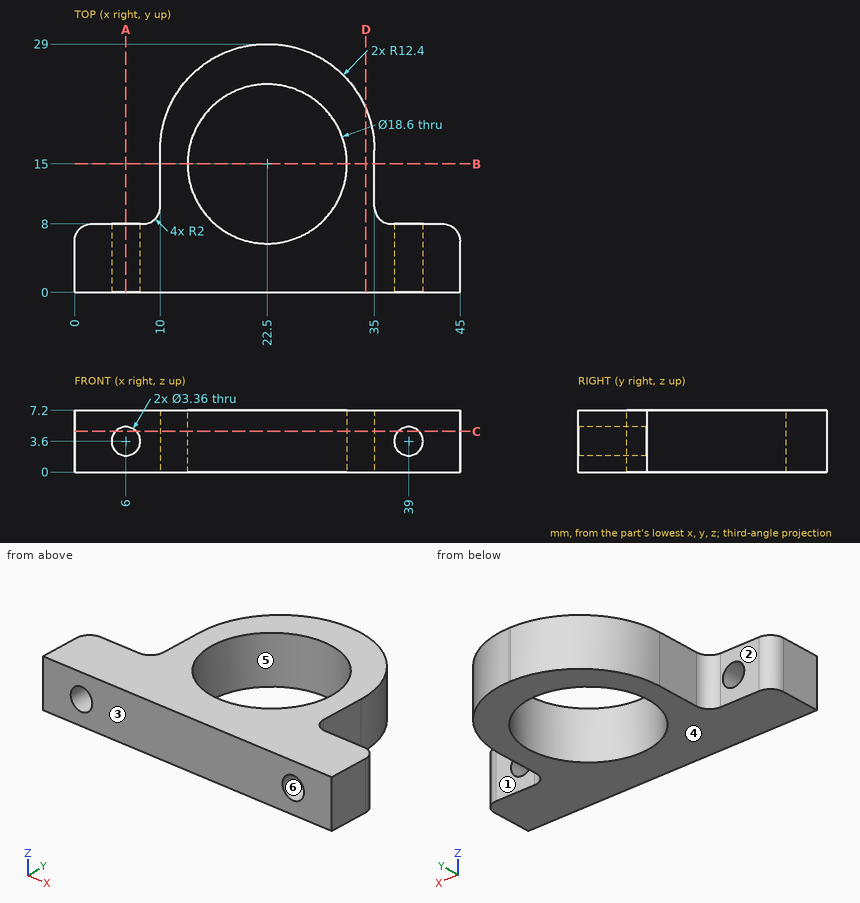
Drawing for the job (mm, zero at the part's lowest x, y, z). A direction names the side the tool comes from. Give positions to 0.01 mm unless a question says otherwise; leave off trailing zeros. Order: outer loops, then holes, each group sorted by start corner. A loop starts at its lowest first (then second) coordinate and runs counter-clockwise, first axis right, second up. Notation, with made-up numbers: (-9.5, -16) - (12.5, -16) arc R21 cw to (12.5, 1) - close; hole circle Ø2 at (-16, -38). An arc over 180 degrees is marked (long way). Use one line per item in the form item = value.
Item 1: Two-plate mould, pull along Z, no slides. Class the marked faces 4, 5 and 6: released by +Z, released by -Z, zero draft, split by the parting line, or undercut.
Solution:
face_4 = released by -Z
face_5 = zero draft
face_6 = undercut
Item 2: Slice it at D-D on x = 34. Give the cut face in (y, z).
Solution:
outline = (0, 0) - (21.48, 0) - (21.48, 7.2) - (0, 7.2) - close
Item 3: Probe probe 1 along Y at (x, z) = (22.5, 4); probe 2 along Z at (x, y) = (6, 3.75); probe 3 along X at (y, z) = (6.75, 4). List the from-to ranges inside material, lowest first. Write a range as from..to.
Solution:
probe_1 = 0..5.7, 24.3..29
probe_2 = 0..1.92, 5.28..7.2
probe_3 = 0.15..4.37, 7.63..18.21, 26.79..37.37, 40.63..44.85
Item 4: Slice it at B-B on y = 15. Give the cut face in (x, z).
Solution:
outline = (10, 0) - (13.2, 0) - (13.2, 7.2) - (10, 7.2) - close; (31.8, 0) - (35, 0) - (35, 7.2) - (31.8, 7.2) - close
Item 5: Pin check, flat tips, straight feed: pin 1 Ø3 at (x, z) = (4.5, 2.5) entering from +Y; pin 2 Ø2 at (x, z) = (37.5, 6) entering from +Y; pin 3 Ø2 at (y, z) = (20.5, 1.5) entering from -X; pin 4 Ø5 at (x, y) = (12, 25) entering from +Z. Stop position of each tip, or through.
Solution:
pin_1 = 8
pin_2 = 8.06
pin_3 = 10.34
pin_4 = 7.2
Item 6: Slice it at C-C on z = 4.75. Give the cut face in (x, y), and give its area (3 significant figures).
Solution:
outline = (0, 0) - (4.78, 0) - (4.78, 8) - (2, 8) arc R2 ccw to (0, 6) - close; (7.22, 0) - (37.78, 0) - (37.78, 8) - (37, 8) arc R2 cw to (35, 10) - (35, 16.6) arc R12.4 ccw to (22.6, 29) - (22.4, 29) arc R12.4 ccw to (10, 16.6) - (10, 10) arc R2 cw to (8, 8) - (7.22, 8) - close; (40.22, 0) - (45, 0) - (45, 6) arc R2 ccw to (43, 8) - (40.22, 8) - close; hole circle Ø18.6 at (22.5, 15)
area = 508 mm2
Item 7: Slice it at A-A on x = 6. Give the cut face in (y, z).
Solution:
outline = (0, 0) - (8, 0) - (8, 1.92) - (0, 1.92) - close; (0, 5.28) - (8, 5.28) - (8, 7.2) - (0, 7.2) - close
Item 8: Which spindle directions (+Z, -Z, +X, -X, +Y, -Y) get a long thin tool onto all of the face, cutting with end or side? Do the marked faces 1, 2 and 3. Say none if no direction does.
Solution:
face_1 = +Z, -Z, +X, +Y
face_2 = +Z, -Z, -X, +Y
face_3 = +Z, -Z, +X, -X, -Y
